Design review of the part built by this model. Coordinates are the model's own, in mm. Face numbers are marked on the shaded views. A direction names the side the tool comes from. Give positions to 0.01 mm unless a question says otherwise; leave off trailing zeros. Order: outer loops, then holes, each group sorted by start corner. A loop starts at its lowest first (then second) coordinate and runs counter-clockwise, first axis right, second up. Notation, with made-up numbers: (41.25, 13) - (92.25, 13) arc R18 ccw to (92.25, 34) - close; hole circle Ø2 at (58, 23.5). An arc over 180 degrees is marked (long way). Write each question's results on one line, items separated by ' | '. Start each with the question number.
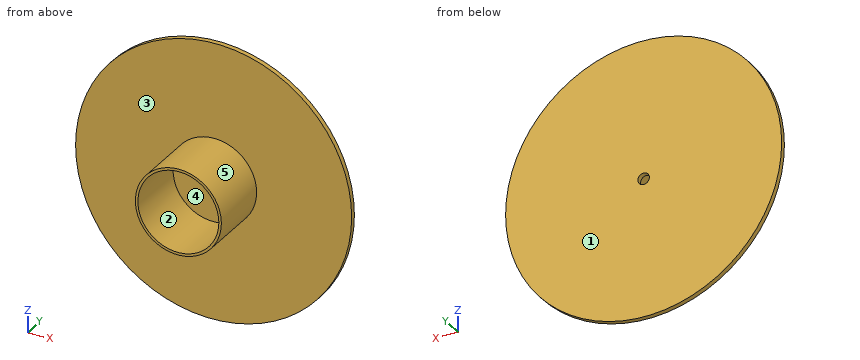
```python
from build123d import *

# Parameters (mm, degrees)
SKETCH1_R           = 76.2
BOSS_EXTRUDE1_DEPTH = 2.76606
SKETCH4_R           = 23.73503
SKETCH4_R_2         = 22.352
BOSS_EXTRUDE3_DEPTH = 35.56
SKETCH5_R           = 3.175
CUT_EXTRUDE1_DEPTH  = 3.76606


with BuildPart() as part:
    # Sketch1 → Boss-Extrude1 (new body)
    with BuildSketch(Plane(origin=(0, 0, 0), x_dir=(1, 0, 0), z_dir=(0, 1, 0))):
        Circle(SKETCH1_R)
    extrude(amount=BOSS_EXTRUDE1_DEPTH)

    # Sketch4 → Boss-Extrude3 (add)
    with BuildSketch(Plane.XZ):
        Circle(SKETCH4_R)
        Circle(SKETCH4_R_2, mode=Mode.SUBTRACT)
    extrude(amount=BOSS_EXTRUDE3_DEPTH)

    # Sketch5 → Cut-Extrude1 (cut, through all)
    with BuildSketch(Plane.XZ):
        Circle(SKETCH5_R)
    extrude(amount=-CUT_EXTRUDE1_DEPTH, mode=Mode.SUBTRACT)


solid = part.part
```
Q1. Insertion check: pin 1 Ø4 at (x, z) = (-17, -48) entering from -Y; pin 2 Ø4 at (x, z) = (0, 0) entering from -Y. Each pin has a flat end and moves straight along its axis. Give the tip position at first contact, or say it passes through.
Q2. Add section B-B (z = 0). Give the boundary of the cut face in (x, y) (3 decimals).
Q3. For line 1 (Z direction, x = 0, y = -26); line 2 (Z direction, x = 0, y = 1.1) (3 decimals); line 3 (Y direction, x = -44.5, z = -7), list the stretches that pass through material, from the lowest coordinate up. Write a range as [from, to].
Q4. Add section A-A (x = 0). Give the boundary of the cut face in (y, z) (3 decimals).
Q5. Add section C-C (y = -28). Give the boundary of the cut face in (x, z).
Q6. Draft analysis for pull direction X (two halves, no side actions). For the marked faces 3, 4 and 5, state which applies: pulls with the +X half, pulls with the -X half, needs draft (parallel to the pull), parting line crosses it, or undercut.
Q7. Machinability: for the marked faces 1 and 2, which of the approach directions +Z, -Z, +X, -X, +Y, -Y give a long, thin tool a straight path to every point of the face, cutting with its end or side? Answer none if there is none.
Q8. Add section D-D (z = 20.5). Give the boundary of the cut face in (x, y).
Verdict:
1) pin 1: stops at y = 0 | pin 2: passes through
2) outline: (-76.2, 0) - (-23.735, 0) - (-23.735, -35.56) - (-22.352, -35.56) - (-22.352, 0) - (-3.175, 0) - (-3.175, 2.766) - (-76.2, 2.766) - close; (3.175, 0) - (22.352, 0) - (22.352, -35.56) - (23.735, -35.56) - (23.735, 0) - (76.2, 0) - (76.2, 2.766) - (3.175, 2.766) - close
3) line 1: z = [-23.74, -22.35], [22.35, 23.74] | line 2: z = [-76.2, -3.175], [3.175, 76.2] | line 3: y = [0, 2.77]
4) outline: (-35.56, -23.735) - (0, -23.735) - (0, -76.2) - (2.766, -76.2) - (2.766, -3.175) - (0, -3.175) - (0, -22.352) - (-35.56, -22.352) - close; (-35.56, 22.352) - (0, 22.352) - (0, 3.175) - (2.766, 3.175) - (2.766, 76.2) - (0, 76.2) - (0, 23.735) - (-35.56, 23.735) - close
5) outline: circle Ø47.47 at (0, 0); hole circle Ø44.7 at (0, 0)
6) face 3: needs draft | face 4: undercut | face 5: parting line crosses it
7) face 1: +Z, -Z, +X, -X, +Y | face 2: -Y
8) outline: (-73.39, 0) - (-11.96, 0) - (-11.96, -35.56) - (-8.91, -35.56) - (-8.91, 0) - (8.91, 0) - (8.91, -35.56) - (11.96, -35.56) - (11.96, 0) - (73.39, 0) - (73.39, 2.77) - (-73.39, 2.77) - close
